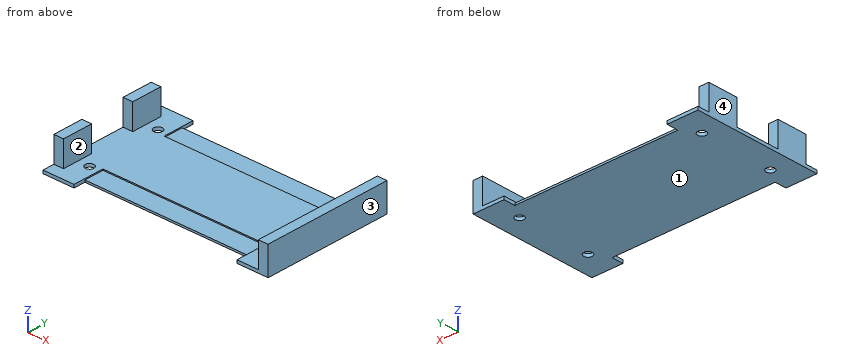
from build123d import *

# Parameters (mm, degrees)
SKETCH1_R           = 1.1
BOSS_EXTRUDE1_DEPTH = 0.8
SKETCH2_W           = 42
SKETCH2_H           = 27
BOSS_EXTRUDE2_DEPTH = 0.5
SKETCH3_W           = 2.5
SKETCH3_H           = 33
SKETCH3_H_2         = 7.8
BOSS_EXTRUDE3_DEPTH = 6.5


with BuildPart() as part:
    # Sketch1 → Boss-Extrude1 (new body)
    with BuildSketch(Plane.XY.offset(-2.3)):
        Polygon((52, -5), (55, -5), (55, 28), (52, 28), (47, 28), (47, 20), (5, 20), (5, 28), (0, 28), (-3, 28), (-3, -5), (0, -5), (5, -5), (5, 3), (47, 3), (47, -5), align=None)
        with Locations((49.5, 2)):
            Circle(SKETCH1_R, mode=Mode.SUBTRACT)
        with Locations((49.5, 21)):
            Circle(SKETCH1_R, mode=Mode.SUBTRACT)
        with Locations((2.5, 2)):
            Circle(SKETCH1_R, mode=Mode.SUBTRACT)
        with Locations((2.5, 21)):
            Circle(SKETCH1_R, mode=Mode.SUBTRACT)
    extrude(amount=BOSS_EXTRUDE1_DEPTH)

    # Sketch2 → Boss-Extrude2 (add)
    with BuildSketch(Plane.XY.offset(-2.3)):
        with Locations((26, 11.5)):
            Rectangle(SKETCH2_W, SKETCH2_H)
    extrude(amount=BOSS_EXTRUDE2_DEPTH)

    # Sketch3 → Boss-Extrude3 (add)
    with BuildSketch(Plane.XY.offset(-1.5)):
        with Locations((53.75, 11.5)):
            Rectangle(SKETCH3_W, SKETCH3_H)
        with Locations((-1.75, 1.9)):
            Rectangle(SKETCH3_W, SKETCH3_H_2)
        with Locations((-1.75, 21.1)):
            Rectangle(SKETCH3_W, SKETCH3_H_2)
    extrude(amount=BOSS_EXTRUDE3_DEPTH)


solid = part.part
Input: part model. Units: mm. Frame: model coordinates. Face numbers are marked on the shaded views. Coordinates: 2 decimals unless noted, no trailing zeros. Write each loop counter-clockwise with the first axis right and the second up, starting at its lowest first coordinate (ties: lowest second). Pieces come first, ordered by that corner, then holes. Notation, with made-up numbers: M 9.5,12.25 L 33.5,12.25 A23 cw 33.5,43.25 Z; hole C -7,55.5 d8. An arc over 180 degrees is marked long. Answer as a JSON object with one key per item and string values. Group by question number.
(1) Mould query, pull axis X, two halves, no side actions, for the marked faces 1, 2, 3 and 4. Classes: pulls with the +X half, pulls with the -X half, needs draft (parallel to the pull), parting line crosses it, or undercut.
(2) Section A-A on z = 2.75. Output: boundary loops of the cut face in (x, y), plus the area to 4 significant figures.
(3) Section D-D on x = 40.5. Output: boundary loops of the cut face in (y, z).
(4) Contact query for flat-ended pins moving along their axis: P1, Ø3, axis at x = -2, z = 0.5, coming from the +Y side; P2, Ø5.5, axis at x = 35.5, y = 0, coming from the +Z side; P3, Ø6, axis at x = 16, y = 1.5, coming from the +Z side; P4, Ø3.5, axis at x = 2.5, y = 21, coming from the -Z side. Output: stop coordinate, or through.
(5) Section C-C on y = 2. Output: boundary loops of the cut face in (x, z), plus the area to 3 significant figures.
(6) Section B-B on x = 49.5. Output: boundary loops of the cut face in (y, z), plus the area to 3 significant figures.
(7) Ray query, line 1 along Y through (x, z) = (49.5, -1.8); line 2 along X through (y, z) = (2, -1); line 3 along Y through (x, z) = (44, -2). Return the intervals inside material, ascending. Write a range as [from, to].
Result set:
{
 "1": {"face 1": "needs draft", "face 2": "undercut", "face 3": "pulls with the +X half", "face 4": "pulls with the -X half"},
 "2": {"outline": "M -3,-2 L -0.5,-2 L -0.5,5.8 L -3,5.8 Z; M -3,17.2 L -0.5,17.2 L -0.5,25 L -3,25 Z; M 52.5,-5 L 55,-5 L 55,28 L 52.5,28 Z", "area": "121.5 mm2"},
 "3": {"outline": "M -2,-2.3 L 25,-2.3 L 25,-1.8 L 20,-1.8 L 20,-1.5 L 3,-1.5 L 3,-1.8 L -2,-1.8 Z"},
 "4": {"P1": "stops at y = 25", "P2": "stops at z = -1.8", "P3": "stops at z = -1.5", "P4": "stops at z = -2.3"},
 "5": {"outline": "M -3,-2.3 L 1.4,-2.3 L 1.4,-1.5 L -0.5,-1.5 L -0.5,5 L -3,5 Z; M 3.6,-2.3 L 48.4,-2.3 L 48.4,-1.5 L 47,-1.5 L 47,-1.8 L 5,-1.8 L 5,-1.5 L 3.6,-1.5 Z; M 50.6,-2.3 L 55,-2.3 L 55,5 L 52.5,5 L 52.5,-1.5 L 50.6,-1.5 Z", "area": "62.8 mm2"},
 "6": {"outline": "M -5,-2.3 L 0.9,-2.3 L 0.9,-1.5 L -5,-1.5 Z; M 3.1,-2.3 L 19.9,-2.3 L 19.9,-1.5 L 3.1,-1.5 Z; M 22.1,-2.3 L 28,-2.3 L 28,-1.5 L 22.1,-1.5 Z", "area": "22.9 mm2"},
 "7": {"line 1": "y = [-5, 0.9], [3.1, 19.9], [22.1, 28]", "line 2": "x = [-3, -0.5], [52.5, 55]", "line 3": "y = [-2, 25]"}
}
